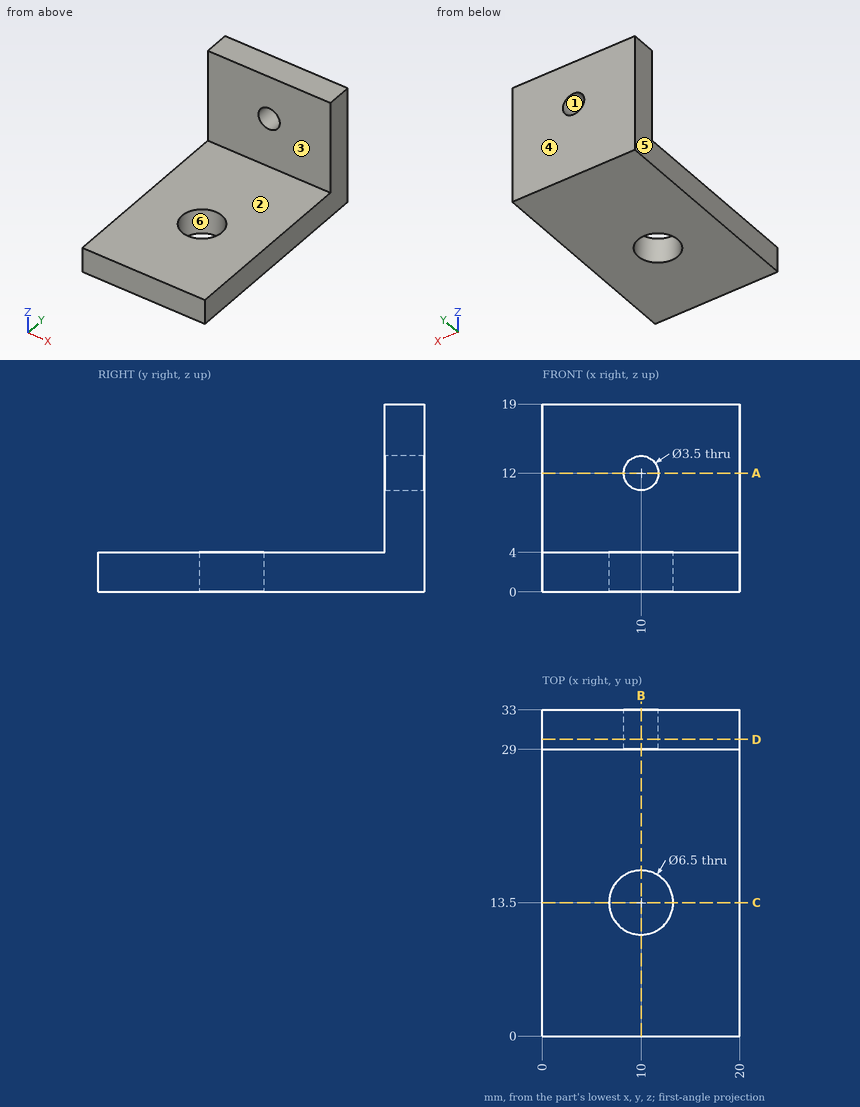
Answer from the drawing. Dimensions are ordinates in mm from the lowest x, y and z of the part. A direction names the side the tool comes from. Round coordinates to 2 decimals unless told otherwise and drop trailing zeros. Order: outer loops, then holes, each group sorted by start corner. A loop starts at its lowest first (then second) coordinate and runs counter-clockwise, first axis right, second up. Notation, with made-up numbers: (-22.5, -30) -> (35.5, -30) arc R19 cw to (35.5, 1) -> close; hole circle Ø5 at (73, -7.5). An arc over 180 degrees is marked (long way). Answer as CSV lines item,"result".
Q1. Which of the six approach directions +Z, -Z, +X, -X, +Y, -Y give full straight-line access (tool end or side, diameter ignored) to the marked faces 1 and 2?
Computed values:
face 1,"+Y, -Y"
face 2,"+Z, +X, -X, -Y"
Q2. For a pull along Y with two mould halves and no side action, classify the marked faces 3, 4, 5 and 6 as +Y half, -Y half, draft (parallel to the pull), parting line (faces both ways), or undercut.
Computed values:
face 3,"-Y half"
face 4,"+Y half"
face 5,"draft"
face 6,"undercut"
Q3. A cutting plane is placed at D-D on y = 30. Determine the outline of the cut face in (x, z).
Computed values:
outline,"(0, 0) -> (20, 0) -> (20, 19) -> (0, 19) -> close; hole circle Ø3.5 at (10, 12)"
Q4. A cutting plane is placed at B-B on x = 10. Determine the outline of the cut face in (y, z).
Computed values:
outline,"(0, 0) -> (10.25, 0) -> (10.25, 4) -> (0, 4) -> close; (16.75, 0) -> (33, 0) -> (33, 10.25) -> (29, 10.25) -> (29, 4) -> (16.75, 4) -> close; (29, 13.75) -> (33, 13.75) -> (33, 19) -> (29, 19) -> close"
Q5. A cutting plane is placed at A-A on z = 12. Determine the outline of the cut face in (x, y).
Computed values:
outline,"(0, 29) -> (8.25, 29) -> (8.25, 33) -> (0, 33) -> close; (11.75, 29) -> (20, 29) -> (20, 33) -> (11.75, 33) -> close"
Q6. Consider line 1 (X direction, y = 31.4, z = 12); line 2 (Y direction, x = 10, z = 3.15); line 3 (Z direction, x = 3.75, y = 7). Determine where each line is inside the solid, lowest interval first. Write a range as from..to.
Computed values:
line 1,"x = 0..8.25, 11.75..20"
line 2,"y = 0..10.25, 16.75..33"
line 3,"z = 0..4"
Q7. Given pin 1 (4.5 mm diameter, centred on x = 10, z = 12, fed in from +Y); pin 2 (7.5 mm diameter, centred on x = 10.5, z = 8, fed in from -Y); pin 3 (8.5 mm diameter, centred on x = 10, y = 13.5, fed in from +Z), each flat-ended and moving along its own axis, determine where each tip first touches the part or whether it passes through.
Computed values:
pin 1,"stops at y = 33"
pin 2,"stops at y = 29"
pin 3,"stops at z = 4"
Q8. A cutting plane is placed at C-C on y = 13.5. Determine the outline of the cut face in (x, z).
Computed values:
outline,"(0, 0) -> (6.75, 0) -> (6.75, 4) -> (0, 4) -> close; (13.25, 0) -> (20, 0) -> (20, 4) -> (13.25, 4) -> close"
